Autodesk Inventor part; units mm, degrees
ref_plane "YZ Plane" through (0, 0, 0) normal (1, 0, 0) x (0, 1, 0)
ref_plane "XZ Plane" through (0, 0, 0) normal (0, 1, 0) x (-1, 0, 0)
ref_plane "XY Plane" through (0, 0, 0) normal (0, 0, 1) x (1, 0, 0)
sketch "Sketch1" plane through (0, 0, 0) normal (0, 1, 0) x (-1, 0, 0)
  line L0 (107.95, 79.375) -> (-107.95, 79.375)
  line L1 (-107.95, 79.375) -> (-107.95, -79.375)
  line L2 (-107.95, -79.375) -> (107.95, -79.375)
  line L3 (107.95, -79.375) -> (107.95, 79.375)
  line L4 (107.95, 79.375) -> (-107.95, -79.375) construction
  line L5 (-107.95, 79.375) -> (107.95, -79.375) construction
  point P0 (0, 0)
  dimension "d0" = 215.9
  dimension "d1" = 158.75
extrude "Extrusion1" add sketch "Sketch1" along normal blind 5
sketch "Sketch2" plane through (0, 5, 0) normal (0, 1, 0) x (1, 0, 0)
  line L0 (107.95, 79.375) -> (-107.95, 79.375)
  line L1 (-107.95, 79.375) -> (-101.6, 79.375)
  line L2 (-101.6, 79.375) -> (-101.6, 73.025)
  line L3 (-101.6, 73.025) -> (-107.95, 73.025)
  line L4 (-107.95, 73.025) -> (-107.95, 79.375)
  line L5 (107.95, 79.375) -> (101.6, 79.375)
  line L6 (101.6, 79.375) -> (101.6, 73.025)
  line L7 (101.6, 73.025) -> (107.95, 73.025)
  line L8 (107.95, 73.025) -> (107.95, 79.375)
  point P0 (0, 0)
  dimension "d4" = 6.35
  dimension "d5" = 6.35
  dimension "d6" = 6.35
  dimension "d7" = 6.35
extrude "Extrusion2" cut sketch "Sketch2" against normal up to next
sketch "Sketch3" plane through (0, 5, 0) normal (0, 1, 0) x (1, 0, 0)
  point P0 (0, 0)
  point P1 (-52.5, 52.5)
  point P2 (-52.5, -52.5)
  point P3 (52.5, -52.5)
  point P4 (52.5, 52.5)
  dimension "d17" = 105
  dimension "d18" = 105
  dimension "d19" = 52.5
  dimension "d20" = 52.5
  dimension "d21" = 105
  dimension "d22" = 52.5
  dimension "d23" = 105
  dimension "d24" = 52.5
hole "Hole1" at (-52.5, 5, -52.5) at (-52.5, 5, 52.5) at (52.5, 5, 52.5) at (52.5, 5, -52.5) direction (0, -1, 0) diameter 6 depth 10.9728 tip angle 118
sketch "Sketch4" plane through (0, 5, 0) normal (0, 1, 0) x (1, 0, 0)
  circle A0 centre (0, 0) radius 69
  dimension "d25" = 138
extrude "Extrusion3" cut sketch "Sketch4" against normal up to next
properties part number "PowerSupplyEncEnds"
CAD build for the part. Positions are in the model's coordinates, mm. A direction names the side the tool comes from. Round coordinates to 2 decimals unless told otherwise and drop trailing zeros. Write each loop counter-clockwise with the first axis right and the second up, starting at its lowest first coordinate (ties: lowest second). Pieces come first, ordered by that corner, then holes. Notation, with made-up numbers: (33, -38) - (72, -38) arc R7 ccw to (72, -31) - close; hole circle Ø11 at (49.5, 60). An arc over 180 degrees is marked (long way). Return JSON: item names as keys, results as strings. Group by question number.
Item 1: 3-axis set-ups, long thin cutter, end or side, ignore diameter. For faces 1 (the face through (105, 3, -73.025)), 2 (the face through (-101.6, 3, -76)), 3 (the face through (-54.53, 2.46, -54.71)): which of +Z, -Z, +X, -X, +Y, -Y reach the whole face in a straight line?
Item 2: Band-saw the part on A-A on y = 1.9. List the corners of the cut face in (x, z) (3 decimals), plus the area to 3 significant figures.
Item 3: Probe probe 1 along Z at (x, y) = (52.5, 3.55) (3 decimals); probe 2 along X at (y, z) = (2.2, -52.5); probe 3 along X at (y, z) = (3.55, 0). List the from-to ranges inside material, lowest first.
Item 4: Mould opens along X. For faces 4 (the face through (50.47, 2.46, -54.71)), 5 (the face through (-105, 3, -73.025)), 6 (the face through (107.95, 2, 4)) say: +X half, -X half, draft (parallel to the pull), parting line (faces both ways), or undercut.
Item 5: Flat gauge pins, fed straight in: pin 1 Ø1.5 at (x, y) = (-103.5, 3.5) entering from -Z (3 decimals); pin 2 Ø2.5 at (y, z) = (2, -76.5) entering from -X; pin 3 Ø7 at (x, z) = (-52.5, -52.5) entering from -Y. Where does each tip first touch, or does it go through?
Item 6: Band-saw the part on B-B on x = 0. List the corners of the cut face in (y, z) (3 decimals), plus the area to 3 significant figures.
Item 7: Band-saw the part on C-C on z = -42.5. List the corners of the cut face in (x, y), plus the area to 3 significant figures.
Item 8: Band-saw the part on D-D on x = 52.5. List the corners of the cut face in (y, z) (3 decimals).
Resolved:
{
 "1": {"face 1": "-Z, +X, +Y, -Y", "face 2": "-Z, -X, +Y, -Y", "face 3": "+Y, -Y"},
 "2": {"outline": "(-107.95, -73.025) - (-101.6, -73.025) - (-101.6, -79.375) - (101.6, -79.375) - (101.6, -73.025) - (107.95, -73.025) - (107.95, 79.375) - (-107.95, 79.375) - close; hole circle Ø138 at (0, 0); hole circle Ø6 at (-52.5, -52.5); hole circle Ø6 at (-52.5, 52.5); hole circle Ø6 at (52.5, -52.5); hole circle Ø6 at (52.5, 52.5)", "area": "19,100 mm²"},
 "3": {"probe 1": "z = -79.375 to -55.5, -49.5 to -44.774, 44.774 to 49.5, 55.5 to 79.375", "probe 2": "x = -107.95 to -55.5, -49.5 to -44.77, 44.77 to 49.5, 55.5 to 107.95", "probe 3": "x = -107.95 to -69, 69 to 107.95"},
 "4": {"face 4": "undercut", "face 5": "draft", "face 6": "+X half"},
 "5": {"pin 1": "stops at z = -73.025", "pin 2": "stops at x = -101.6", "pin 3": "stops at y = 0"},
 "6": {"outline": "(0, -79.375) - (5, -79.375) - (5, -69) - (0, -69) - close; (0, 69) - (5, 69) - (5, 79.375) - (0, 79.375) - close", "area": "104 mm²"},
 "7": {"outline": "(-107.95, 0) - (-54.36, 0) - (-54.36, 5) - (-107.95, 5) - close; (54.36, 0) - (107.95, 0) - (107.95, 5) - (54.36, 5) - close", "area": "536 mm²"},
 "8": {"outline": "(0, -79.375) - (5, -79.375) - (5, -55.5) - (0, -55.5) - close; (0, -49.5) - (5, -49.5) - (5, -44.774) - (0, -44.774) - close; (0, 44.774) - (5, 44.774) - (5, 49.5) - (0, 49.5) - close; (0, 55.5) - (5, 55.5) - (5, 79.375) - (0, 79.375) - close"}
}
